Source: CAD feature listing. Evaluate the final solid. Frame: model axes, mm. A direction names the side the tool comes from. Coordinates: 2 decimals unless noted, no trailing zeros. Loops run counter-clockwise (first coordinate to the right, second up) from the corner with the lowest first, then second, coordinate; pieces in that order, holes last. Notation, with made-up numbers: M 43.5,42 L 98.5,42 A22 cw 98.5,58 Z; hole C 20.5,25.25 d8. An arc over 180 degrees is marked long. One line per question, with ' | ' between items. Start each with the question number.
1. Ray query, probe 1 along Z at (x, y) = (-224.5, 33.45) (3 decimals); probe 2 along Z at (x, y) = (-195.5, 34.5). Return the intervals inside material, ascending.
2. Pin query (flat end, axial travel): P1, Ø1.6, axis at x = -198.5, y = 34.5, coming from the +Z side (3 decimals); P2, Ø1, axis at y = 35, z = -8.5, coming from the +X side; P3, Ø1.6, axis at y = 34, z = -1.5, coming from the +X side. Return the tip coordinate at first contact, or that it passes through.
3. Section query A-A, the plane y = 34.1. Output: boundary loops of the cut face in (x, z) (3 decimals).
4. Section query B-B, the plane x = -225. Output: boundary loops of the cut face in (y, z) (3 decimals), and give its area (3 significant figures).
5. Mould query, pull axis Z, two halves, no side actions, for faces 5 (the flat face through (-219, 34, -100.673)), 6 (the flat face through (-190.313, 34, -99)), 7 (the flat face through (-198, 34, -3.175)). Classes: pulls with the +Z half, pulls with the -Z half, needs draft (parallel to the pull), parting line crosses it, or undercut.
6. Section query C-C, the plane x = -192. Output: boundary loops of the cut face in (y, z), and give its area (3 significant figures).
7. Access query for faces 1 (the flat face through (-196.663, 34, -5)), 2 (the flat face through (-214, 34, -3.175)), 3 (the flat face through (-215.713, 34, -102)), 4 (the flat face through (-187, 34, -97.498)). Directions: +Z, -Z, +X, -X, +Y, -Y. A direction counts if a zero-diameter tool reaches every point of the face in a straight line with its end or side. Return the directions, or none.
```python
from build123d import *

# Parameters (mm, degrees)
SKETCH1_W           = 44.45
SKETCH1_H           = 3.175
BOSS_EXTRUDE1_DEPTH = 107.022511
CUT_EXTRUDE1_DEPTH  = 253.262317967


with BuildPart() as part:
    # Sketch1 → Boss-Extrude1 (new body)
    with BuildSketch(Plane.XY):
        with Locations((-206.187737343, 34.464226646)):
            Rectangle(SKETCH1_W, SKETCH1_H)
    extrude(amount=-BOSS_EXTRUDE1_DEPTH)

    # Sketch2 → Cut-Extrude1 (cut, through all)
    with BuildSketch(Plane(origin=(0, 36.051726646, 0), x_dir=(1, 0, 0), z_dir=(0, 1, 0))):
        Polygon((-228.412737343, 107.022511379), (-222.062737343, 107.022511379), (-215.712737343, 107.022511379), (-212.537737343, 107.022511379), (-212.537737343, 103.847511379), (-215.712737343, 103.847511379), (-215.712737343, 100.672511379), (-222.062737343, 100.672511379), (-222.062737343, 97.497511379), (-228.412737343, 97.497511379), align=None)
        Polygon((-183.962737343, 107.022511379), (-190.312737343, 107.022511379), (-196.662737343, 107.022511379), (-199.837737343, 107.022511379), (-199.837737343, 103.847511379), (-196.662737343, 103.847511379), (-196.662737343, 100.672511379), (-190.312737343, 100.672511379), (-190.312737343, 97.497511379), (-183.962737343, 97.497511379), align=None)
        Polygon((-228.412737343, 0), (-222.062737343, 0), (-215.712737343, 0), (-212.537737343, 0), (-212.537737343, 3.175), (-215.712737343, 3.175), (-215.712737343, 6.35), (-222.062737343, 6.35), (-222.062737343, 9.525), (-228.412737343, 9.525), align=None)
        Polygon((-183.962737343, 0), (-190.312737343, 0), (-196.662737343, 0), (-199.837737343, 0), (-199.837737343, 3.175), (-196.662737343, 3.175), (-196.662737343, 6.35), (-190.312737343, 6.35), (-190.312737343, 9.525), (-183.962737343, 9.525), align=None)
    extrude(amount=-CUT_EXTRUDE1_DEPTH, mode=Mode.SUBTRACT)


solid = part.part
```
Taken from the geometry:
1) probe 1: -97.498 to -9.525 | probe 2: -100.67 to -6.35
2) P1: z = -3.175 | P2: x = -190.31 | P3: x = -199.84
3) outline: M -228.413,-97.498 L -222.063,-97.498 L -222.063,-100.673 L -215.713,-100.673 L -215.713,-103.848 L -212.538,-103.848 L -212.538,-107.023 L -199.838,-107.023 L -199.838,-103.848 L -196.663,-103.848 L -196.663,-100.673 L -190.313,-100.673 L -190.313,-97.498 L -183.963,-97.498 L -183.963,-9.525 L -190.313,-9.525 L -190.313,-6.35 L -196.663,-6.35 L -196.663,-3.175 L -199.838,-3.175 L -199.838,0 L -212.538,0 L -212.538,-3.175 L -215.713,-3.175 L -215.713,-6.35 L -222.063,-6.35 L -222.063,-9.525 L -228.413,-9.525 Z
4) outline: M 32.877,-97.498 L 36.052,-97.498 L 36.052,-9.525 L 32.877,-9.525 Z | area: 279 mm^2
5) face 5: pulls with the -Z half | face 6: needs draft | face 7: pulls with the +Z half
6) outline: M 32.88,-100.67 L 36.05,-100.67 L 36.05,-6.35 L 32.88,-6.35 Z | area: 299 mm^2
7) face 1: +Z, +X, +Y, -Y | face 2: +Z, -X, +Y, -Y | face 3: -Z, -X, +Y, -Y | face 4: -Z, +X, +Y, -Y
